Autodesk Inventor part; units mm, degrees
ref_plane "YZ Plane" through (0, 0, 0) normal (1, 0, 0) x (0, 1, 0)
ref_plane "XZ Plane" through (0, 0, 0) normal (0, 1, 0) x (-1, 0, 0)
ref_plane "XY Plane" through (0, 0, 0) normal (0, 0, 1) x (1, 0, 0)
sketch "スケッチ1" plane through (0, 0, 0) normal (0, 1, 0) x (-1, 0, 0)
  line L0 (12, 32) -> (-12, 32)
  line L1 (-12, 32) -> (-12, -32)
  line L2 (-12, -32) -> (12, -32)
  line L3 (12, -32) -> (12, 32)
  line L4 (12, 32) -> (-12, -32) construction
  line L5 (-12, 32) -> (12, -32) construction
  line L6 (8.25, 25) -> (-8.25, 25)
  line L7 (-8.25, 25) -> (-8.25, -25)
  line L8 (-8.25, -25) -> (8.25, -25)
  line L9 (8.25, -25) -> (8.25, 25)
  line L10 (8.25, 25) -> (-8.25, -25) construction
  line L11 (-8.25, 25) -> (8.25, -25) construction
  point P0 (0, 0)
  dimension "d0" = 24
  dimension "d1" = 64
  dimension "d2" = 16.5
  dimension "d3" = 50
extrude "押し出し1" add sketch "スケッチ1" along normal blind 2
sketch "スケッチ2" plane through (0, 2, 0) normal (0, 1, 0) x (1, 0, 0)
  point P0 (0, 0)
fillet "フィレット1" radius 3 4 edges at (-12, 1, 32) (12, 1, 32) (12, 1, -32) (-12, 1, -32)
properties part number "bottom"
Model file for the job. Use its own axes, mm. A direction names the side the tool comes from. Give positions to 0.01 mm unless a question says otherwise; leave off trailing zeros. Write each loop counter-clockwise with the first axis right and the second up, starting at its lowest first coordinate (ties: lowest second). Pieces come first, ordered by that corner, then holes. Notation, with made-up numbers: (53, 84) -> (107, 84) arc R20 ccw to (107, 93) -> close; hole circle Ø1 at (46.5, 56). An arc over 180 degrees is marked (long way). Write item = value, one per line.
(1) Tool access for faces 1 (the face through (11.14, 1.01, -31.1)), 2 (the face through (-8.25, 1, 0)): list every direction of +Z, -Z, +X, -X, +Y, -Y with a clear straight run to the whole face (end or side of a thin tool).
Determined:
face_1 = -Z, +X, +Y, -Y
face_2 = +Y, -Y
(2) Probe line 1 along Z through (x, y) = (2.5, 1); line 2 along X through (y, z) = (0.3, -4); line 3 along Z through (x, y) = (-10.5, 0.5). List the from-to ranges inside material, lowest first.
Determined:
line_1 = -32 to -25, 25 to 32
line_2 = -12 to -8.25, 8.25 to 12
line_3 = -31.6 to 31.6
(3) Flat gauge pin, fed straight in: P1, Ø10, axis at x = -3, z = 6.5, coming from the -Y side. Where does the tip first touch, or does it go through?
Determined:
P1 = through
(4) Slice it at B-B, the plane y = 0.45. Give the cut face in (x, z).
Determined:
outline = (-12, -29) arc R3 ccw to (-9, -32) -> (9, -32) arc R3 ccw to (12, -29) -> (12, 29) arc R3 ccw to (9, 32) -> (-9, 32) arc R3 ccw to (-12, 29) -> close; hole (-8.25, -25) -> (8.25, -25) -> (8.25, 25) -> (-8.25, 25) -> close
(5) Mould opens along X. For faces 3 (the face through (8.25, 1, 0)), 4 (the face through (-12, 1, 0)), 5 (the face through (12, 1, 0)) say: released by +X, released by -X, zero draft, split by the parting line, or undercut.
Determined:
face_3 = undercut
face_4 = released by -X
face_5 = released by +X
(6) Slice it at A-A, the plane z = 22. Give the cut face in (x, y), then the cut area to 3 significant figures.
Determined:
outline = (-12, 0) -> (-8.25, 0) -> (-8.25, 2) -> (-12, 2) -> close; (8.25, 0) -> (12, 0) -> (12, 2) -> (8.25, 2) -> close
area = 15.0 mm2
(7) Slice it at C-C, the plane x = -3. Give the cut face in (y, z), then the cut area to 3 significant figures.
Determined:
outline = (0, -32) -> (2, -32) -> (2, -25) -> (0, -25) -> close; (0, 25) -> (2, 25) -> (2, 32) -> (0, 32) -> close
area = 28.0 mm2
